Autodesk Inventor part; units mm, degrees
ref_plane "YZ Plane" through (0, 0, 0) normal (1, 0, 0) x (0, 1, 0)
ref_plane "XZ Plane" through (0, 0, 0) normal (0, 1, 0) x (-1, 0, 0)
ref_plane "XY Plane" through (0, 0, 0) normal (0, 0, 1) x (1, 0, 0)
sketch "Szkic1" plane through (0, 0, 0) normal (0, 1, 0) x (-1, 0, 0)
  circle A0 centre (0, 0) radius 5.5
  dimension "d0" = 11
extrude "Wyciągnięcie proste1" add sketch "Szkic1" along normal blind 45
sketch "Szkic2" plane through (0, 45, 0) normal (0, 1, 0) x (1, 0, 0)
  circle A0 centre (0, 0) radius 6
  dimension "d3" = 12
extrude "Wyciągnięcie proste2" add sketch "Szkic2" against normal blind 2
sketch "Szkic3" plane through (0, 45, 0) normal (0, 1, 0) x (1, 0, 0)
  point P0 (0, 0)
  point P1 (0, 0)
hole "Otwór1" at (0, 45, 0) direction (0, -1, 0) diameter 6.5 end through all
properties part number "Jack_srodek"
The model under review builds one solid part; all positions refer to its coordinate system, in mm. Give positions to 0.01 mm unless a question says otherwise; leave off trailing zeros. Write each loop counter-clockwise with the first axis right and the second up, starting at its lowest first coordinate (ties: lowest second). Pieces come first, ordered by that corner, then holes. Notation, with made-up numbers: M 42.25,-20.5 L 81.25,-20.5 A22 ccw 81.25,-0.5 Z; hole C 66,51 d11. An arc over 180 degrees is marked long. Write item = value, one per line. Start each with the question number.
Q1. We need section A-A (z = 0). State the section outline as (x, y) points, plus the area to 4 significant figures.
Q2. We need section C-C (y = 34). State the section outline as (x, z) points.
Q3. Mouldability with a two-part tool opening along X and no side actions: class faces 1 (the face through (3, 43, 5)), 2 (the face through (1.978, 22.185, -2.579)), 3 (the face through (1.19, 21.2, 5.37)) as released by +X, released by -X, zero draft, split by the parting line, or undercut.
Q4. We need section D-D (z = -4.5). State the section outline as (x, y) points, plus the area to 3 significant figures.
Q5. Clearance check with flat-ended pins moving along their axes: pin 1 (6 mm diameter, centred on x = -4.5, z = 5, fed in from -Y); pin 2 (4 mm diameter, centred on x = -4.5, y = 27, fed in from -Z); pin 3 (6 mm diameter, centred on x = 1.5, y = 39, fed in from -Z); pin 4 (3 mm diameter, centred on y = 17, z = 4, fed in from -X). State where each tip first meets the part, or that it passes through.
Q6. We need section B-B (x = 0). State the section outline as (y, z) points.
Q7. For line 1 (X direction, y = 25.5, z = 0); line 2 (Z direction, x = 2, y = 18), list the stretches that pass through material, from the lowest coordinate up.
Result set:
q1.outline = M -6,43 L -5.5,43 L -5.5,0 L -3.25,0 L -3.25,45 L -6,45 Z; M 3.25,0 L 5.5,0 L 5.5,43 L 6,43 L 6,45 L 3.25,45 Z
q1.area = 204.5 mm2
q2.outline = C 0,0 d11; hole C 0,0 d6.5
q3.face_1 = zero draft
q3.face_2 = undercut
q3.face_3 = split by the parting line
q4.outline = M -3.97,43 L -3.16,43 L -3.16,0 L 3.16,0 L 3.16,43 L 3.97,43 L 3.97,45 L -3.97,45 Z
q4.area = 288 mm2
q5.pin_1 = 0
q5.pin_2 = -4.9
q5.pin_3 = -5.5
q5.pin_4 = -4.9
q6.outline = M 0,-5.5 L 43,-5.5 L 43,-6 L 45,-6 L 45,-3.25 L 0,-3.25 Z; M 0,3.25 L 45,3.25 L 45,6 L 43,6 L 43,5.5 L 0,5.5 Z
q7.line_1 = -5.5 to -3.25, 3.25 to 5.5
q7.line_2 = -5.12 to -2.56, 2.56 to 5.12
